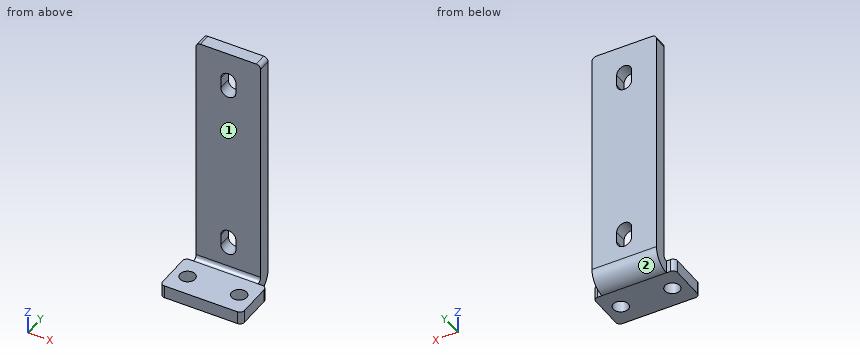
```python
from build123d import *

# Parameters (mm, degrees)
CROQUIS1_W             = 19
CROQUIS1_H             = 10
CROQUIS1_R             = 1.75
BRIDA_BASE1_DEPTH      = 3
BRIDA_DE_ARISTA1_DEPTH = 15
CORTAR_EXTRUIR1_REACH  = 61.85
REDONDEO1_R            = 1


# Sheet-metal steps are written as plain solids
with BuildPart() as part:
    # Croquis1 → Brida base1 (new body)
    with BuildSketch(Plane.XY):
        with Locations((9.5, -5)):
            Rectangle(CROQUIS1_W, CROQUIS1_H)
        with Locations((3.5, -5)):
            Circle(CROQUIS1_R, mode=Mode.SUBTRACT)
        with Locations(Location((15.5, -5, 0), (0, 0, 180))):
            Circle(CROQUIS1_R, mode=Mode.SUBTRACT)
    extrude(amount=-BRIDA_BASE1_DEPTH)

    # Brida de arista1 section (across the edge) → Brida de arista1 (add)
    with BuildSketch(Plane(origin=(17, 1, 0), x_dir=(0, -1, 0), z_dir=(-1, 0, 0))):
        with BuildLine():
            Line((-3, 1), (-3, 55))
            Line((-3, 55), (0, 55))
            Line((0, 55), (0, 1))
            ThreePointArc((0, 1), (0.292893219, 0.292893219), (1, 0))
            Line((1, 0), (1, -3))
            ThreePointArc((1, -3), (-1.828427125, -1.828427125), (-3, 1))
        make_face()
    extrude(amount=BRIDA_DE_ARISTA1_DEPTH)

    # Croquis9 → Cortar-Extruir1 (cut, up to next)
    with BuildSketch(Plane(origin=(0, 4, 0), x_dir=(1, 0, 0), z_dir=(0, 1, 0)), mode=Mode.PRIVATE) as cortar_extruir1_sk1:
        with BuildLine():
            Line((7.75, -8.25), (7.75, -5.75))
            ThreePointArc((7.75, -5.75), (9.5, -4), (11.25, -5.75))
            Line((11.25, -5.75), (11.25, -8.25))
            ThreePointArc((11.25, -8.25), (9.5, -10), (7.75, -8.25))
        make_face()
    cortar_extruir1_tool1 = extrude(cortar_extruir1_sk1.sketch, amount=-CORTAR_EXTRUIR1_REACH, mode=Mode.PRIVATE) & part.part
    # Croquis9 → Cortar-Extruir1 (cut, up to next)
    with BuildSketch(Plane(origin=(0, 4, 0), x_dir=(1, 0, 0), z_dir=(0, 1, 0)), mode=Mode.PRIVATE) as cortar_extruir1_sk2:
        with BuildLine():
            Line((7.75, -48.25), (7.75, -45.75))
            ThreePointArc((7.75, -45.75), (9.5, -44), (11.25, -45.75))
            Line((11.25, -45.75), (11.25, -48.25))
            ThreePointArc((11.25, -48.25), (9.5, -50), (7.75, -48.25))
        make_face()
    cortar_extruir1_tool2 = extrude(cortar_extruir1_sk2.sketch, amount=-CORTAR_EXTRUIR1_REACH, mode=Mode.PRIVATE) & part.part
    add(cortar_extruir1_tool1.solids().sort_by_distance((9.5, 4, 7))[0], mode=Mode.SUBTRACT)
    add(cortar_extruir1_tool2.solids().sort_by_distance((9.5, 4, 47))[0], mode=Mode.SUBTRACT)

    # Redondeo1
    redondeo1_edges = [part.edges().sort_by_distance(p)[0] for p in [
        (19, -10, -1.5),
        (0, -10, -1.5),
        (19, 0, -1.5),
        (0, 0, -1.5),
        (17, 2.5, 55),
        (2, 2.5, 55),
    ]]
    fillet(redondeo1_edges, radius=REDONDEO1_R)


solid = part.part
```
Check sheet for the modelled part. Datum: model origin and axes. Units: mm. Face numbers are marked on the shaded views. A direction names the side the tool comes from. Round coordinates to 2 decimals unless told otherwise and drop trailing zeros. Loops run counter-clockwise (first coordinate to the right, second up) from the corner with the lowest first, then second, coordinate; pieces in that order, holes last. Notation, with made-up numbers: (68.5, 43.5) - (102.5, 43.5) arc R16 ccw to (102.5, 69.5) - close; hole circle Ø1 at (22, 65). An arc over 180 degrees is marked (long way). Write item = value, one per line. Start each with the question number.
Q1. Section check A-A (x = 9.5). Record the boundary of the cut face in (y, z).
Q2. Section check B-B (x = 6.25). Record the boundary of the cut face in (y, z).
Q3. Depth check by flat-ended pin: P1, Ø3, axis at x = 15.5, y = -5, coming from the -Z side; P2, Ø2, axis at x = 10.5, z = 39.5, coming from the -Y side; P3, Ø2, axis at y = 3, z = 47.5, coming from the -X side; P4, Ø2, axis at y = 3, z = 47, coming from the +X side. Enter the tip coordinate at first touch or a pass-through.
Q4. Section check C-C (y = 2). Record the boundary of the cut face in (x, z).
Q5. Section check D-D (z = 11.5). Record the boundary of the cut face in (x, y), plus the area to 3 significant figures.
Q6. Access from +Z, -Z, +X, -X, +Y, -Y to the whole of each face (thin tool, end or side, straight path). Record for the marked faces 1 and 2.
Q7. Thickness scan on L1, parallel to Z at x = 9.5, y = 2.75; L2, parallel to Y at x = 6.75, z = 51.5; L3, parallel to X at y = 3.5, z = 31.5. Record the ranges inside material, lowest first.
Derived:
q1.outline = (-10, -3) - (0, -3) arc R4 ccw to (4, 1) - (4, 4) - (1, 4) - (1, 1) arc R1 cw to (0, 0) - (-10, 0) - close; (1, 10) - (4, 10) - (4, 44) - (1, 44) - close; (1, 50) - (4, 50) - (4, 55) - (1, 55) - close
q2.outline = (-10, -3) - (0, -3) arc R4 ccw to (4, 1) - (4, 55) - (1, 55) - (1, 1) arc R1 cw to (0, 0) - (-10, 0) - close
q3.P1 = through
q3.P2 = 1
q3.P3 = 2
q3.P4 = 17
q4.outline = (2, -2.46) - (17, -2.46) - (17, 54) arc R1 ccw to (16, 55) - (3, 55) arc R1 ccw to (2, 54) - close; hole (7.75, 5.75) arc R1.75 ccw to (11.25, 5.75) - (11.25, 8.25) arc R1.75 ccw to (7.75, 8.25) - close; hole (7.75, 45.75) arc R1.75 ccw to (11.25, 45.75) - (11.25, 48.25) arc R1.75 ccw to (7.75, 48.25) - close
q5.outline = (2, 1) - (17, 1) - (17, 4) - (2, 4) - close
q5.area = 45.0 mm^2
q6.face_1 = +Z, +X, -X, -Y
q6.face_2 = -Z, +X, -X, +Y
q7.L1 = -1.9 to 4, 10 to 44, 50 to 55
q7.L2 = 1 to 4
q7.L3 = 2 to 17
